```python
from build123d import *

# Parameters (mm, degrees)
SKETCH1_R               = 796.925
SKETCH1_R_2             = 746.125
BOSS_EXTRUDE1_DEPTH     = 18.25625
CUT_EXTRUDE2_DEPTH      = 1128.169996901
SKETCH4_W               = 88.9
SKETCH4_H               = 44.45
SKETCH4_W_2             = 44.45
SKETCH4_H_2             = 88.9
BOSS_EXTRUDE2_DEPTH     = 18.25625
SKETCH10_W              = 88.9
SKETCH10_H              = 1.5875
SKETCH10_W_2            = 1.5875
SKETCH10_H_2            = 88.9
CUT_EXTRUDE3_DEPTH      = 1128.169996901
SKETCH11_W              = 1.240607087
SKETCH11_H              = 42.8625
SKETCH11_W_2            = 42.8625
SKETCH11_H_2            = 1.240607087
CUT_EXTRUDE4_DEPTH      = 1128.169996901
BOSS_EXTRUDE4_DEPTH     = 18.25625
CUT_EXTRUDE5_DEPTH      = 1126.415744032
F_1_4_CLEARANCE_HOLE3_D = 6.7564
F_1_4_CLEARANCE_HOLE1_D = 6.7564
CUT_EXTRUDE6_DEPTH      = 1126.415744032
FILLET4_R               = 3.3782


with BuildPart() as part:
    # Sketch1 → Boss-Extrude1 (new body)
    with BuildSketch(Plane(origin=(0, 0, 0), x_dir=(1, 0, 0), z_dir=(0, 1, 0))):
        with Locations(Location((0, 0, 0), (0, 0, 270))):
            Circle(SKETCH1_R)
        with Locations(Location((0, 0, 0), (0, 0, 270))):
            Circle(SKETCH1_R_2, mode=Mode.SUBTRACT)
    extrude(amount=BOSS_EXTRUDE1_DEPTH)

    # Sketch3 → Cut-Extrude2 (cut, through all)
    with BuildSketch(Plane(origin=(0, 18.25625, 0), x_dir=(1, 0, 0), z_dir=(0, 1, 0))):
        with BuildLine():
            Line((-796.925, 0), (0, 0))
            Line((0, 0), (0, -796.925))
            ThreePointArc((0, -796.925), (563.511071597, 563.511071597), (-796.925, 0))
        make_face()
    extrude(amount=-CUT_EXTRUDE2_DEPTH, mode=Mode.SUBTRACT)

    # Sketch4 → Boss-Extrude2 (add)
    with BuildSketch(Plane(origin=(0, 18.25625, 0), x_dir=(1, 0, 0), z_dir=(0, 1, 0))):
        with Locations((-752.475, -22.225)):
            Rectangle(SKETCH4_W, SKETCH4_H)
        with Locations((-22.225, -752.475)):
            Rectangle(SKETCH4_W_2, SKETCH4_H_2)
    extrude(amount=-BOSS_EXTRUDE2_DEPTH)

    # Sketch10 → Cut-Extrude3 (cut, through all)
    with BuildSketch(Plane(origin=(0, 18.25625, 0), x_dir=(1, 0, 0), z_dir=(0, 1, 0))):
        with Locations((-752.475, -0.79375)):
            Rectangle(SKETCH10_W, SKETCH10_H)
        with Locations((-0.79375, -752.475)):
            Rectangle(SKETCH10_W_2, SKETCH10_H_2)
    extrude(amount=-CUT_EXTRUDE3_DEPTH, mode=Mode.SUBTRACT)

    # Sketch11 → Cut-Extrude4 (cut, through all)
    with BuildSketch(Plane(origin=(0, 18.25625, 0), x_dir=(1, 0, 0), z_dir=(0, 1, 0))):
        with Locations((-796.304696457, -23.01875)):
            Rectangle(SKETCH11_W, SKETCH11_H)
        with Locations((-23.01875, -796.304696457)):
            Rectangle(SKETCH11_W_2, SKETCH11_H_2)
    extrude(amount=-CUT_EXTRUDE4_DEPTH, mode=Mode.SUBTRACT)

    # Sketch12 → Boss-Extrude4 (add, through all)
    with BuildSketch(Plane(origin=(0, 18.25625, 0), x_dir=(1, 0, 0), z_dir=(0, 1, 0))):
        with BuildLine():
            Line((-45.731111071, -708.025), (-79.575539683, -741.869428612))
            ThreePointArc((-79.575539683, -741.869428612), (-62.030076286, -743.542053458), (-44.45, -744.799780562))
            Line((-44.45, -744.799780562), (-44.45, -708.025))
            Line((-44.45, -708.025), (-45.731111071, -708.025))
        make_face()
        with BuildLine():
            Line((-708.025, -45.731111071), (-741.869428612, -79.575539683))
            ThreePointArc((-741.869428612, -79.575539683), (-743.542053458, -62.030076286), (-744.799780562, -44.45))
            Line((-744.799780562, -44.45), (-708.025, -44.45))
            Line((-708.025, -44.45), (-708.025, -45.731111071))
        make_face()
    extrude(amount=-BOSS_EXTRUDE4_DEPTH)

    # Sketch14 → Cut-Extrude5 (cut, through all)
    with BuildSketch(Plane.XZ):
        Polygon((-166.462625141, 960.559518053), (42.242196456, 751.854696456), (-751.854696456, -42.242196456), (-960.559518053, 166.462625141), (-949.662084803, 177.360058391), (-747.606322079, -24.695704333), (24.695704333, 747.606322079), (-177.360058391, 949.662084803), align=None)
    extrude(amount=-CUT_EXTRUDE5_DEPTH, mode=Mode.SUBTRACT)

    # 1/4 Clearance Hole3 (through all)
    with Locations(Plane(origin=(0, 18.25625, 0), x_dir=(1, 0, 0), z_dir=(0, 1, 0))):
        with Locations((-752.09645014, -22.450640303), (-22.450640303, -752.09645014)):
            Hole(F_1_4_CLEARANCE_HOLE3_D / 2)

    # 1/4 Clearance Hole1 (through all)
    with Locations(Plane(origin=(0, 18.25625, 0), x_dir=(1, 0, 0), z_dir=(0, 1, 0))):
        with Locations((-747.606322079, -197.565634664), (-545.550559355, -545.550559355), (-197.565634664, -747.606322079)):
            Hole(F_1_4_CLEARANCE_HOLE1_D / 2)

    # Sketch19 → Cut-Extrude6 (cut, through all)
    with BuildSketch(Plane(origin=(0, 18.25625, 0), x_dir=(1, 0, 0), z_dir=(0, 1, 0))):
        Polygon((-774.547090442, -2.24506403), (-720.665553716, -2.24506403), (-747.606322079, 24.695704333), align=None)
        Polygon((-708.317701549, -14.592916197), (-708.025, -14.885617746), (-708.025, -45.731111071), (-708.317701549, -46.02381262), align=None)
        Polygon((-14.885617746, -708.025), (-45.731111071, -708.025), (-46.02381262, -708.317701549), (-14.592916197, -708.317701549), align=None)
        Polygon((24.695704333, -747.606322079), (-2.24506403, -774.547090442), (-2.24506403, -720.665553716), align=None)
    extrude(amount=-CUT_EXTRUDE6_DEPTH, mode=Mode.SUBTRACT)

    # Fillet4
    fillet4_edges = [part.edges().sort_by_distance(p)[0] for p in [
        (-79.575539683, 9.128125, 741.869428612),
        (-741.869428612, 9.128125, 79.575539683),
    ]]
    fillet(fillet4_edges, radius=FILLET4_R)


solid = part.part
```
Here's how the part is built. I have some questions about the finished solid (model axes, mm). A direction names the side the tool comes from. Round coordinates to 2 decimals unless told otherwise and drop trailing zeros. Write each loop counter-clockwise with the first axis right and the second up, starting at its lowest first coordinate (ties: lowest second). Pieces come first, ordered by that corner, then holes.
Q1. Will these pins go through, and if not, where does the flat tip stop? P1, Ø1.5, axis at y = 12, z = 609, coming from the +X side; P2, Ø5.5, axis at y = 5, z = 32, coming from the +X side; P3, Ø2, axis at y = 3.5, z = 393.5, coming from the -X side; P4, Ø6, axis at x = -545.55, z = 545.55, coming from the -Y side.
Q2. If we mould it in two halves opening along Z, with no side actions, what happens to faces 4 (the flat face through (-785.3, 9, 13)), 5 (the flat face through (-548, 18.256, 515)), 6 (the flat face through (-724.295, 9.256, 62.001))? For each: +Z half, -Z half, draft (parallel to the pull), parting line (faces both ways), or undercut.
Q3. Which directions (+Z, -Z, +X, -X, +Y, -Y) give clear straight access to the entire face, cutting with the end or side of a thin tool? Please do faces 1 (the flat face through (-12.7, 9, 785)), 2 (the flat face through (-31, 9, 708.318)), 3 (the flat face through (-62.001, 9.256, 724.295)).
Q4. If we section it at C-C on x = -438: Write out the boundary of the cut face in (y, z).
Q5. If we section it at A-A on y = 12.25: Write out the boundary of the cut face in (x, z) (3 decimals), plus the area to 3 significant figures.
Q6. Please list where these lines run through material, in increasing order: probe 1 along Z at (x, y) = (-42.5, 3.75); probe 2 along Z at (x, y) = (-130, 4.75); probe 3 along X at (y, z) = (12, 666).
Q7. If we section it at B-B on z = 571.5: Write out the boundary of the cut face in (x, y).
Answer below:
1. P1: stops at x = -430.01
1. P2: stops at x = -708.32
1. P3: stops at x = -693.57
1. P4: passes through
2. face 4: -Z half
2. face 5: draft
2. face 6: undercut
3. face 1: +Z, +X, +Y, -Y
3. face 2: -Z, +X, +Y, -Y
3. face 3: -Z, +Y, -Y
4. outline: (0, 604.04) - (18.26, 604.04) - (18.26, 665.77) - (0, 665.77) - close
5. outline: (-795.684, 23.382) - (-774.547, 2.245) - (-720.666, 2.245) - (-708.318, 14.593) - (-708.318, 46.024) - (-740.725, 78.431) arc R3.378 cw to (-741.695, 81.188) arc R746.125 cw to (-81.188, 741.695) arc R3.378 cw to (-78.431, 740.725) - (-46.024, 708.318) - (-14.593, 708.318) - (-2.245, 720.666) - (-2.245, 774.547) - (-23.382, 795.684) - (-44.45, 795.684) arc R796.925 ccw to (-795.684, 44.45) - close; hole circle Ø6.756 at (-752.096, 22.451); hole circle Ø6.756 at (-747.606, 197.566); hole circle Ø6.756 at (-545.551, 545.551); hole circle Ø6.756 at (-197.566, 747.606); hole circle Ø6.756 at (-22.451, 752.096)
5. area: 65,000 mm2
6. probe 1: z = 708.32 to 795.68
6. probe 2: z = 734.71 to 786.25
6. probe 3: x = -437.65 to -336.37
7. outline: (-555.41, 0) - (-479.68, 0) - (-479.68, 18.26) - (-555.41, 18.26) - close
